```python
from build123d import *

# Parameters (mm, degrees)
SKETCH1_R           = 30.4
BOSS_EXTRUDE1_DEPTH = 15
BOSS_EXTRUDE7_DEPTH = 15
FILLET2_R           = 5
BOSS_EXTRUDE8_DEPTH = 15


with BuildPart() as part:
    # Sketch1 → Boss-Extrude1 (new body)
    with BuildSketch(Plane(origin=(0, 0, 0), x_dir=(1, 0, 0), z_dir=(0, 1, 0))):
        with Locations(Location((0, 0, 0), (0, 0, 270))):
            Circle(SKETCH1_R)
    extrude(amount=BOSS_EXTRUDE1_DEPTH)

    # Sketch2 → Boss-Extrude7 (add)
    with BuildSketch(Plane.XY):
        with BuildLine():
            Line((12.281826966, 50.600114208), (-18.575808631, 50.600114208))
            Line((-18.575808631, 50.600114208), (-18.575808631, 15))
            Line((-18.575808631, 15), (27.386025108, 15))
            Line((27.386025108, 15), (27.386025108, 0))
            Line((27.386025108, 0), (35, 0))
            ThreePointArc((35, 0), (62.733044116, 42.851436224), (12.281826966, 50.600114208))
        make_face()
    extrude(amount=BOSS_EXTRUDE7_DEPTH)

    # Fillet2
    fillet2_edges = [part.edges().sort_by_distance(p)[0] for p in [
        (12.281826966, 50.600114208, 7.5),
        (-18.575808631, 50.600114208, 7.5),
        (-29.393755023, 15, -7.756749685),
    ]]
    fillet(fillet2_edges, radius=FILLET2_R)

    # Sketch4 → Boss-Extrude8 (add)
    with BuildSketch(Plane(origin=(0, 0, 0), x_dir=(-1, 0, 0), z_dir=(0, 0, -1))):
        with BuildLine():
            Line((-43.716283143, 50.097045256), (-35, 35))
            ThreePointArc((-35, 35), (-32.7, 34.383716857), (-31.016283143, 32.7))
            Line((-31.016283143, 32.7), (-13.583716857, 32.7))
            ThreePointArc((-13.583716857, 32.7), (-5, 30.4), (-13.583716857, 28.1))
            Line((-13.583716857, 28.1), (-31.016283143, 28.1))
            ThreePointArc((-31.016283143, 28.1), (-32.7, 26.416283143), (-35, 25.8))
            Line((-35, 25.8), (-43.716283143, 10.702954744))
            ThreePointArc((-43.716283143, 10.702954744), (-50, 4.419237886), (-47.7, 13.002954744))
            Line((-47.7, 13.002954744), (-38.983716857, 28.1))
            ThreePointArc((-38.983716857, 28.1), (-39.6, 30.4), (-38.983716857, 32.7))
            Line((-38.983716857, 32.7), (-47.7, 47.797045256))
            ThreePointArc((-47.7, 47.797045256), (-50, 56.380762114), (-43.716283143, 50.097045256))
        make_face()
    extrude(amount=BOSS_EXTRUDE8_DEPTH)


solid = part.part
```
Verification items for the finished model (mm, model axes). A direction names the side the tool comes from. Round coordinates to 2 decimals unless told otherwise and drop trailing zeros. Loops run counter-clockwise (first coordinate to the right, second up) from the corner with the lowest first, then second, coordinate; pieces in that order, holes last. Notation, with made-up numbers: (-8, 75) -> (41, 75) arc R14 cw to (41, 100) -> close; hole circle Ø9 at (23, 18). An arc over 180 degrees is marked (long way). Answer as a JSON object with one key per item and string values.
Q1. Go/stop test with flat-tipped pins: P1, Ø5, axis at y = 10, z = -8, coming from the +X side; P2, Ø18, axis at x = 18.5, y = 44, coming from the +Z side; P3, Ø10, axis at y = 7.5, z = 7.5, coming from the -X side. Record where each tip stops, or that it passes through.
Data:
{"P1": "stops at x = 52.3", "P2": "stops at z = 15", "P3": "stops at x = -30.3"}
Q2. Draft check along Y on faces 5 (the flat face through (43.4, 20.45, -7.4)), 6 (the flat face through (34, 31, -15)), 7 (the cylindrical face through (-17.072, 49.174, 7.605)). Enter one of: pulls with the +Y half, pulls with the -Y half, needs draft (parallel to the pull), parting line crosses it, or undercut.
Data:
{"face 5": "undercut", "face 6": "needs draft", "face 7": "pulls with the +Y half"}
Q3. Access from +Z, -Z, +X, -X, +Y, -Y to the whole of each face (thin tool, end or side, straight path). Record for faces 1 (the cylindrical face through (50.144, 56.294, -7.395)), 2 (the cylindrical face through (32.73, 34.4, -7.4)), 3 (the flat face through (-18.576, 31, 7)), 4 (the flat face through (0.4, 15, -0.4)).
Data:
{"face 1": "-Z", "face 2": "-Z, +Y", "face 3": "+Z, -Z, -X, +Y", "face 4": "-X"}
Q4. Section check A-A (x = 0). Record the boundary of the cut face in (y, z), then the cut area to 3 significant figures.
Data:
{"outline": "(0, -30.4) -> (10, -30.4) arc R5 ccw to (15, -25.4) -> (15, 0) -> (50.6, 0) -> (50.6, 15) -> (15, 15) -> (15, 25.4) arc R5 ccw to (10, 30.4) -> (0, 30.4) -> close", "area": "1,440 mm2"}
Q5. Section check B-B (y = 30.4). Record the boundary of the cut face in (x, z).
Data:
{"outline": "(-18.58, 0) -> (5, 0) -> (5, -15) -> (39.6, -15) -> (39.6, 0) -> (65.4, 0) -> (65.4, 15) -> (-18.58, 15) -> close"}
Q6. Scan lines: line 1 (Y direction, x = 18, z = -5); line 2 (Y direction, x = -9, z = 23.5). Record each from-to range of solid material in increasing order. Write a range as from..to.
Data:
{"line 1": "y = 0..15, 28.1..32.7", "line 2": "y = 0..15"}
Q7. Section check C-C (x = 37.5). Record the boundary of the cut face in (y, z), then the cut area to 3 significant figures.
Data:
{"outline": "(0.1, 0) -> (21.47, 0) -> (21.47, -15) -> (39.33, -15) -> (39.33, 0) -> (60.7, 0) -> (60.7, 15) -> (0.1, 15) -> close", "area": "1,180 mm2"}
